The model under review builds one solid part; all positions refer to its coordinate system, in mm. A direction names the side the tool comes from. Coordinates: 2 decimals unless noted, no trailing zeros. Use a Markdown table: item, result. Add a question column.
1) Clearance check with flat-ended pins moving along their axes: pin 1 (1.5 mm diameter, centred on x = -9, z = 1.5, fed in from +Y); pin 2 (1.5 mm diameter, centred on y = -12, z = 1.5, fed in from -X); pin 3 (0.9 mm diameter, centred on x = -6, z = 2, fed in from -Y). State where each tip first meets the part, or that it passes through.
2) To check wall thickness, follow L1, parallel to Y at x = -8.75, z = 0.9; L2, parallel to Y at x = -3.75, z = 2.05; L3, parallel to X at y = 62.5, z = 0.7 (3 decimals). State the ranges of each line that lie inside material, in increasing order. Write a range as [from, to].
3) The part is to be moulded in two halves that separate along X. For faces 5 (the flat face through (5, -51, 1)), 6 (the flat face through (-5, 10, 3)), 7 (the flat face through (-1, -45.5, 1)), say which applies: pulls with the +X half, pulls with the -X half, needs draft (parallel to the pull), parting line crosses it, or undercut.
4) For faces 1 (the flat face through (-7, -47, 1)), 2 (the flat face through (-8, 67, 1)), 3 (the flat face through (5, 26, 1)), 4 (the flat face through (-10, -44, 1)), list the 3-axis set-ups (+Z, -Z, +X, -X, +Y, -Y) from which the entire face can be reached by the end or side of a thin tool; tool diameter is ignored.
5) Add section A-A, the plane z = 2.45. Give the number of separate pieces and of enclosed holes in the cut face, and give its area (3 significant figures).
```python
from build123d import *

# Parameters (mm, degrees)
CROQUIS1_W              = 10
CROQUIS1_H              = 3
SALIENTE_EXTRUIR1_DEPTH = 3


with BuildPart() as part:
    # Croquis1 → Saliente-Extruir1 (new body)
    with BuildSketch(Plane.XY):
        with BuildLine():
            Line((-0.5, 63), (0, 63))
            Line((0, 63), (0, 60))
            Line((0, 60), (-0.5, 60))
            Line((-0.5, 60), (-9.5, 60))
            Line((-9.5, 60), (-10, 60))
            Line((-10, 60), (-10, 63))
            Line((-10, 63), (-9.5, 63))
            Line((-9.5, 63), (-7, 63))
            Line((-7, 63), (-7, 67))
            Line((-7, 67), (-10, 67))
            Line((-10, 67), (-10, 70))
            Line((-10, 70), (-15, 70))
            Line((-15, 70), (-15, 67.405747627))
            ThreePointArc((-15, 67.405747627), (-14.929306729, 67.036438809), (-14.727221995, 66.719345288))
            add(Edge.make_bspline(
                [(-14.727221995, 57.280654712), (-13.242407332, 58.853769808), (-11.757592668, 62), (-13.242407332, 65.146230192), (-14.727221995, 66.719345288)],
                knots=[0.028065471, 0.028065471, 0.028065471, 0.028065471, 0.5, 0.971934529, 0.971934529, 0.971934529, 0.971934529], degree=3))
            ThreePointArc((-14.727221995, 57.280654712), (-14.929306729, 56.963561191), (-15, 56.594252373))
            Line((-15, 56.594252373), (-15, 54.181314171))
            ThreePointArc((-15, 54.181314171), (-14.9841425, 54.003934523), (-14.937072921, 53.832180471))
            add(Edge.make_bspline(
                [(-14.937072921, 53.832180471), (-13.31235764, 49.471453647), (-11.68764236, 40.75), (-13.31235764, 32.028546353), (-14.937072921, 27.667819529)],
                knots=[0.006332812, 0.006332812, 0.006332812, 0.006332812, 0.5, 0.993667188, 0.993667188, 0.993667188, 0.993667188], degree=3))
            ThreePointArc((-14.937072921, 27.667819529), (-14.9841425, 27.496065477), (-15, 27.318685829))
            Line((-15, 27.318685829), (-15, 24.567654138))
            ThreePointArc((-15, 24.567654138), (-14.997723384, 24.500214919), (-14.990903903, 24.433082766))
            add(Edge.make_bspline(
                [(-14.990903903, -48.933082766), (-13.330301301, -36.70538851), (-11.669698699, -12.25), (-13.330301301, 12.20538851), (-14.990903903, 24.433082766)],
                knots=[0.000910439, 0.000910439, 0.000910439, 0.000910439, 0.5, 0.999089561, 0.999089561, 0.999089561, 0.999089561], degree=3))
            ThreePointArc((-14.990903903, -48.933082766), (-14.997723384, -49.000214919), (-15, -49.067654138))
            Line((-15, -49.067654138), (-15, -51.701381229))
            Line((-15, -51.701381229), (-15, -52))
            Line((-15, -52), (-10, -52))
            Line((-10, -52), (-10, -49))
            Line((-10, -49), (-7, -49))
            Line((-7, -49), (-7, -45.5))
            Line((-7, -45.5), (-9.5, -45.5))
            Line((-9.5, -45.5), (-10, -45.5))
            Line((-10, -45.5), (-10, -42.5))
            Line((-10, -42.5), (-9.5, -42.5))
            Line((-9.5, -42.5), (-0.5, -42.5))
            Line((-0.5, -42.5), (0, -42.5))
            Line((0, -42.5), (0, -45.5))
            Line((0, -45.5), (-0.5, -45.5))
            Line((-0.5, -45.5), (-3, -45.5))
            Line((-3, -45.5), (-3, -49))
            Line((-3, -49), (0, -49))
            Line((0, -49), (0, -52))
            Line((0, -52), (5, -52))
            Line((5, -52), (5, -51.701381229))
            Line((5, -51.701381229), (5, -49.067654138))
            ThreePointArc((5, -49.067654138), (4.997723384, -49.000214919), (4.990903903, -48.933082766))
            add(Edge.make_bspline(
                [(4.990903903, -48.933082766), (3.330301301, -36.70538851), (1.669698699, -12.25), (3.330301301, 12.20538851), (4.990903903, 24.433082766)],
                knots=[0.000910439, 0.000910439, 0.000910439, 0.000910439, 0.5, 0.999089561, 0.999089561, 0.999089561, 0.999089561], degree=3))
            ThreePointArc((4.990903903, 24.433082766), (4.997723384, 24.500214919), (5, 24.567654138))
            Line((5, 24.567654138), (5, 27.318685829))
            ThreePointArc((5, 27.318685829), (4.9841425, 27.496065477), (4.937072921, 27.667819529))
            add(Edge.make_bspline(
                [(4.937072921, 53.832180471), (3.31235764, 49.471453647), (1.68764236, 40.75), (3.31235764, 32.028546353), (4.937072921, 27.667819529)],
                knots=[0.006332812, 0.006332812, 0.006332812, 0.006332812, 0.5, 0.993667188, 0.993667188, 0.993667188, 0.993667188], degree=3))
            ThreePointArc((4.937072921, 53.832180471), (4.9841425, 54.003934523), (5, 54.181314171))
            Line((5, 54.181314171), (5, 56.594252373))
            ThreePointArc((5, 56.594252373), (4.929306729, 56.963561191), (4.727221995, 57.280654712))
            add(Edge.make_bspline(
                [(4.727221995, 66.719345288), (3.242407332, 65.146230192), (1.757592668, 62), (3.242407332, 58.853769808), (4.727221995, 57.280654712)],
                knots=[0.028065471, 0.028065471, 0.028065471, 0.028065471, 0.5, 0.971934529, 0.971934529, 0.971934529, 0.971934529], degree=3))
            ThreePointArc((4.727221995, 66.719345288), (4.929306729, 67.036438809), (5, 67.405747627))
            Line((5, 67.405747627), (5, 70))
            Line((5, 70), (0, 70))
            Line((0, 70), (0, 67))
            Line((0, 67), (-3, 67))
            Line((-3, 67), (-3, 63))
            Line((-3, 63), (-0.5, 63))
        make_face()
        with Locations((-5, 26)):
            Rectangle(CROQUIS1_W, CROQUIS1_H, mode=Mode.SUBTRACT)
        with Locations((-5, 55.5)):
            Rectangle(CROQUIS1_W, CROQUIS1_H, mode=Mode.SUBTRACT)
    extrude(amount=SALIENTE_EXTRUIR1_DEPTH)


solid = part.part
```
From the geometry:
| question | item | result |
|---|---|---|
| 1 | pin 1 | stops at y = 67 |
| 1 | pin 2 | stops at x = -12.5 |
| 1 | pin 3 | stops at y = -42.5 |
| 2 | L1 | y = [-49, -45.5], [-42.5, 24.5], [27.5, 54], [57, 60], [63, 67] |
| 2 | L2 | y = [-42.5, 24.5], [27.5, 54], [57, 60] |
| 2 | L3 | x = [-12.525, -10], [0, 2.525] |
| 3 | face 5 | pulls with the +X half |
| 3 | face 6 | needs draft |
| 3 | face 7 | undercut |
| 4 | face 1 | +Z, -Z, -Y |
| 4 | face 2 | +Z, -Z, +Y |
| 4 | face 3 | +Z, -Z, +X, +Y, -Y |
| 4 | face 4 | +Z, -Z |
| 5 | separate pieces | 1 |
| 5 | enclosed holes | 2 |
| 5 | area | 1,860 mm^2 |
